Verification items for the finished model (mm, model axes). A direction names the side the tool comes from. Give positions to 0.01 mm unless a question says otherwise; leave off trailing zeros. Loops run counter-clockwise (first coordinate to the right, second up) from the corner with the lowest first, then second, coordinate; pieces in that order, holes last. Notation, with made-up numbers: (-24.5, 8) - (26.5, 8) arc R23 ccw to (26.5, 29) - close; hole circle Ø10 at (55.5, -35.5). An arc over 180 degrees is marked (long way). One line per item, written item: value. Start each with the question number.
1. Sectioned sample at C-C (x = -46.5). Record the cut outline in (y, z).
2. Mould release check, pull along Y, two halves, no side actions. Record for faces 3 (the flat face through (19, 0, 15)), 4 (the flat face through (18.655, 2.733, 19.801)), 5 (the cylindrical face through (25.705, 11.827, 5.376)): pulls with the +Y half, pulls with the -Y half, needs draft (parallel to the pull), parting line crosses it, or undercut.
3. Sectioned sample at D-D (z = 19.25). Record the cut outline in (x, y).
4. Sectioned sample at B-B (x = 25). Record the cut outline in (y, z).
5. Scan lines: L1, parallel to X at y = 15, z = 6.8; L2, parallel to Y at x = 25, z = 1.9; L3, parallel to X at y = 14, z = 3.25. Record each from-to range of solid material in increasing order. Write a range as [from, to].
6. Sectioned sample at A-A (y = 15). Record the cut outline in (x, z).
7. Gauge pin test, flat ends, axial feed: pin 1 (3 mm diameter, centred on x = -33.5, y = 21, fed in from +Z); pin 2 (10 mm diameter, centred on x = 37, y = 20.5, fed in from -Z); pin 3 (5 mm diameter, centred on x = 25, y = 15, fed in from +Z); pin 4 (6 mm diameter, centred on y = 21, z = 12, fed in from +X). Record the tip position at first contact, or that the pin passes through.
8. Access from +Z, -Z, +X, -X, +Y, -Y to the whole of each face (thin tool, end or side, straight path). Record for faces 1 (the flat face through (-65, 11, 6)), 2 (the flat face through (23.6, 13.6, 2.5)).
from build123d import *

# Parameters (mm, degrees)
BOSS_EXTRUDE1_DEPTH  = 100
M3_CLEARANCE_HOLE1_D = 3.4
SKETCH4_R            = 3.25
CUT_EXTRUDE1_DEPTH   = 108.964114408
BOSS_EXTRUDE2_DEPTH  = 65


with BuildPart() as part:
    # Sketch1 → Boss-Extrude1 (new body)
    with BuildSketch(Plane(origin=(0, 0, 0), x_dir=(0, 0, -1), z_dir=(1, 0, 0))):
        Polygon((0, 0), (0, 30), (-5, 30), (-9.312388631, 5.54322876), (-30, 0), align=None)
    extrude(amount=BOSS_EXTRUDE1_DEPTH)

    # M3 Clearance Hole1 (through all)
    with Locations(Plane(origin=(0, 0, 0), x_dir=(-1, 0, 0), z_dir=(0, 0, -1))):
        with Locations((-25, 15), (-75, 15)):
            Hole(M3_CLEARANCE_HOLE1_D / 2)

    # Sketch4 → Cut-Extrude1 (cut, through all)
    with BuildSketch(Plane(origin=(0, 0, 2.5), x_dir=(-1, 0, 0), z_dir=(0, 0, -1))):
        with Locations((-75, 15)):
            Circle(SKETCH4_R)
        with Locations((-25, 15)):
            Circle(SKETCH4_R)
    extrude(amount=-CUT_EXTRUDE1_DEPTH, mode=Mode.SUBTRACT)

    # Sketch6 → Boss-Extrude2 (add)
    with BuildSketch(Plane.ZY):
        Polygon((0, 0), (30, 0), (9.312388631, 5.54322876), (5, 30), (0, 30), align=None)
    extrude(amount=BOSS_EXTRUDE2_DEPTH)


solid = part.part
Results are:
1. outline: (0, 0) - (30, 0) - (30, 5) - (5.54, 9.31) - (0, 30) - close
2. face 3: pulls with the -Y half
2. face 4: pulls with the +Y half
2. face 5: undercut
3. outline: (-65, 0) - (100, 0) - (100, 2.88) - (-65, 2.88) - close
4. outline: (0, 0) - (13.3, 0) - (13.3, 2.5) - (11.75, 2.5) - (11.75, 8.22) - (5.54, 9.31) - (0, 30) - close; (16.7, 0) - (30, 0) - (30, 5) - (18.25, 7.07) - (18.25, 2.5) - (16.7, 2.5) - close
5. L1: x = [-65, 21.75], [28.25, 71.75], [78.25, 100]
5. L2: y = [0, 13.3], [16.7, 30]
5. L3: x = [-65, 21.91], [28.09, 71.91], [78.09, 100]
6. outline: (-65, 0) - (23.3, 0) - (23.3, 2.5) - (21.75, 2.5) - (21.75, 7.64) - (-65, 7.64) - close; (26.7, 0) - (73.3, 0) - (73.3, 2.5) - (71.75, 2.5) - (71.75, 7.64) - (28.25, 7.64) - (28.25, 2.5) - (26.7, 2.5) - close; (76.7, 0) - (100, 0) - (100, 7.64) - (78.25, 7.64) - (78.25, 2.5) - (76.7, 2.5) - close
7. pin 1: stops at z = 6.85
7. pin 2: stops at z = 0
7. pin 3: stops at z = 2.5
7. pin 4: passes through
8. face 1: +Z, -Z, -X, +Y, -Y
8. face 2: +Z
